Work out the finished part from the listing and answer in its coordinate system (mm). A direction names the side the tool comes from. Round coordinates to 2 decimals unless told otherwise and drop trailing zeros. Write each loop counter-clockwise with the first axis right and the second up, starting at its lowest first coordinate (ties: lowest second). Pieces come first, ordered by that corner, then holes.
1. Find section B-B (z = -16). Write down the section's boundary in (x, y).
2. Straight lines are drawn through the part: probe 1 along X at (y, z) = (9.5, -54); probe 2 along Y at (x, z) = (6, -50.75); probe 3 along Z at (x, y) = (12.5, -9.5). For each, find the intervals that lie inside material, in ascending order.
3. Flat-ended cylindrical pins translate along their axes: pin 1 Ø2.5 at (x, y) = (19, 9.5) entering from +Z; pin 2 Ø12.5 at (x, z) = (12, -13.5) entering from +Y; pin 3 Ø5.5 at (x, y) = (17, 9) entering from +Z. Find the tip coordinate at first contact, or state that the pin passes through.
4. A tool of negligible diameter and unlimited length cuts with its end or side. For faces 1 (the face through (10.976, -6.409, -16.632)), 2 (the face through (12, 10, -49)), from which of +Z, -Z, +X, -X, +Y, -Y can it reach the whole face along a straight path? Write none if from no direction.
5. Find section C-C (x = 19). Write down the section's boundary in (y, z), and give its area (3 significant figures).
6. Determine the mould class of faces 3 (the face through (25, -4, -27)), 4 (the face through (19.29, 7.27, -52.13)), 5 (the face through (12, 19, -52)) for opening direction X: pulls with the +X half, pulls with the -X half, needs draft (parallel to the pull), parting line crosses it, or undercut.
7. Find section D-D (y = 9.5). Write down the section's boundary in (x, z).
8. Find section A-A (x = 12.5). Write down the section's boundary in (y, z).
```python
from build123d import *

# Parameters (mm, degrees)
F1_DEPTH       = 25
F3_D           = 4.4958
F3_CSINK_D     = 9.1186
F3_CSINK_ANGLE = 82
F5_D           = 3.3
F6_T1_DEPTH    = 40
F6_T3_DEPTH    = 47


# Not quite as in the source:
# - a fillet or chamfer that OpenCascade refuses, or shapes differently, is made with other operations: its cross-section is extruded or revolved along the edge and cut away or added


with BuildPart() as f1:
    # F0 (on Right) → F1 (new body)
    with BuildSketch(Plane.YZ):
        Polygon((-13, -58), (19, -58), (19, -49), (0, -49), (0, 0), (-13, 0), align=None)
    extrude(amount=F1_DEPTH)

    # F3 (through all)
    with Locations(Plane(origin=(0, 0, -58), x_dir=(1, 0, 0), z_dir=(0, 0, -1))):
        with Locations((6, -9.5), (19, -9.5)):
            CounterSinkHole(F3_D / 2, F3_CSINK_D / 2, counter_sink_angle=F3_CSINK_ANGLE)

    # F5 (through all)
    with Locations(Plane.XZ.offset(13)):
        with Locations((12.5, -16)):
            Hole(F5_D / 2)

    # F6: fillet of radius 3 on 4 edges, made by hand

    # F6_s2 → F6_t1 (cut)
    with BuildSketch(Plane.YZ.offset(-7.5)):
        with BuildLine():
            ThreePointArc((-10, -58), (-12.1213203436, -57.1213203436), (-13, -55))
            Line((-13, -55), (-13, -58))
            Line((-13, -58), (-10, -58))
        make_face()
        with BuildLine():
            ThreePointArc((16, -58), (18.1213203436, -57.1213203436), (19, -55))
            Line((19, -55), (19, -58))
            Line((19, -58), (16, -58))
        make_face()
    extrude(amount=F6_T1_DEPTH, mode=Mode.SUBTRACT)

    # F6_s4 → F6_t3 (cut)
    with BuildSketch(Plane.XZ.offset(-26.5)):
        with BuildLine():
            ThreePointArc((22, -58), (24.1213203436, -57.1213203436), (25, -55))
            Line((25, -55), (25, -58))
            Line((25, -58), (22, -58))
        make_face()
        with BuildLine():
            ThreePointArc((3, -58), (0.8786796564, -57.1213203436), (0, -55))
            Line((0, -55), (0, -58))
            Line((0, -58), (3, -58))
        make_face()
    extrude(amount=F6_T3_DEPTH, mode=Mode.SUBTRACT)


solid = f1.part
```
Worked answers:
1. outline: (0, -13) - (10.85, -13) - (10.85, 0) - (0, 0) - close; (14.15, -13) - (25, -13) - (25, 0) - (14.15, 0) - close
2. probe 1: x = 0 to 3.75, 8.25 to 16.75, 21.25 to 25
2. probe 2: y = -13 to 7.25, 11.75 to 19
2. probe 3: z = -58 to -17.65, -14.35 to 0
3. pin 1: passes through
3. pin 2: stops at y = 0
3. pin 3: stops at z = -49
4. face 1: +Y, -Y
4. face 2: +Z, +X, -X, +Y
5. outline: (-13, -55) arc R3 ccw to (-10, -58) - (4.94, -58) - (7.25, -55.34) - (7.25, -49) - (0, -49) - (0, 0) - (-13, 0) - close; (11.75, -55.34) - (14.06, -58) - (16, -58) arc R3 ccw to (19, -55) - (19, -49) - (11.75, -49) - close
5. area: 875 mm2
6. face 3: pulls with the +X half
6. face 4: undercut
6. face 5: needs draft
7. outline: (0, -55) arc R3 ccw to (1.7, -57.7) - (3.75, -55.34) - (3.75, -49) - (0, -49) - close; (8.25, -55.34) - (10.56, -58) - (14.44, -58) - (16.75, -55.34) - (16.75, -49) - (8.25, -49) - close; (21.25, -55.34) - (23.3, -57.7) arc R3 ccw to (25, -55) - (25, -49) - (21.25, -49) - close
8. outline: (-13, -55) arc R3 ccw to (-10, -58) - (16, -58) arc R3 ccw to (19, -55) - (19, -49) - (0, -49) - (0, -17.65) - (-13, -17.65) - close; (-13, -14.35) - (0, -14.35) - (0, 0) - (-13, 0) - close
